from build123d import *

# Parameters (mm, degrees)
SKETCH1_W                = 33
SKETCH1_H                = 33
BOSS_EXTRUDE1_DEPTH      = 33
SKETCH2_W                = 21
SKETCH2_H                = 21
CUT_EXTRUDE1_DEPTH       = 58.15767665
SKETCH3_W                = 21
SKETCH3_H                = 21
CUT_EXTRUDE2_DEPTH       = 58.15767665
SKETCH4_W                = 21
SKETCH4_H                = 21
CUT_EXTRUDE3_DEPTH       = 58.15767665
SKETCH5_R                = 3.05
CUT_EXTRUDE4_DEPTH       = 58.15767665
SKETCH6_R                = 3.05
CUT_EXTRUDE5_DEPTH       = 58.15767665
SKETCH7_R                = 3.05
CUT_EXTRUDE6_DEPTH       = 58.15767665
FILLET1_R                = 6
CHAMFER1_START           = -1
CHAMFER1_OUTLINE_W       = 16
CHAMFER1_OUTLINE_H       = 18
CHAMFER1_DEPTH           = 6.773502692
BOSS_EXTRUDE3_DEPTH      = 8
BOSS_EXTRUDE3_DEPTH_BACK = 10
SKETCH9_W                = 18
SKETCH9_H                = 18
CHAMFER2_SIZE            = 6
FILLET2_R                = 1.25
SKETCH10_R               = 6
BOSS_EXTRUDE4_DEPTH      = 10
SKETCH11_R               = 6
BOSS_EXTRUDE5_DEPTH      = 10
SKETCH12_R               = 6
BOSS_EXTRUDE6_DEPTH      = 10
FILLET3_R                = 2
FILLET4_R                = 2.5


with BuildPart() as part:
    # Sketch1 → Boss-Extrude1 (new body)
    with BuildSketch(Plane(origin=(0, 0, 0), x_dir=(1, 0, 0), z_dir=(0, 1, 0))):
        with Locations((16.5, -16.5)):
            Rectangle(SKETCH1_W, SKETCH1_H)
    extrude(amount=BOSS_EXTRUDE1_DEPTH)

    # Sketch2 → Cut-Extrude1 (cut, through all)
    with BuildSketch(Plane.XY.offset(33)):
        with Locations((22.5, 22.5)):
            Rectangle(SKETCH2_W, SKETCH2_H)
    extrude(amount=-CUT_EXTRUDE1_DEPTH, mode=Mode.SUBTRACT)

    # Sketch3 → Cut-Extrude2 (cut, through all)
    with BuildSketch(Plane.XZ):
        with Locations((22.5, 22.5)):
            Rectangle(SKETCH3_W, SKETCH3_H)
    extrude(amount=-CUT_EXTRUDE2_DEPTH, mode=Mode.SUBTRACT)

    # Sketch4 → Cut-Extrude3 (cut, through all)
    with BuildSketch(Plane.ZY):
        with Locations((22.5, 22.5)):
            Rectangle(SKETCH4_W, SKETCH4_H)
    extrude(amount=-CUT_EXTRUDE3_DEPTH, mode=Mode.SUBTRACT)

    # Sketch5 → Cut-Extrude4 (cut, through all)
    with BuildSketch(Plane.ZY):
        with Locations((27, 6)):
            Circle(SKETCH5_R)
        with Locations((6, 18)):
            Circle(SKETCH5_R)
    extrude(amount=-CUT_EXTRUDE4_DEPTH, mode=Mode.SUBTRACT)

    # Sketch6 → Cut-Extrude5 (cut, through all)
    with BuildSketch(Plane.XZ):
        with Locations(Location((6, 18, 0), (0, 0, 270))):
            Circle(SKETCH6_R)
        with Locations(Location((27, 6, 0), (0, 0, 270))):
            Circle(SKETCH6_R)
    extrude(amount=-CUT_EXTRUDE5_DEPTH, mode=Mode.SUBTRACT)

    # Sketch7 → Cut-Extrude6 (cut, through all)
    with BuildSketch(Plane(origin=(0, 0, 0), x_dir=(-1, 0, 0), z_dir=(0, 0, -1))):
        with Locations((-18, 6)):
            Circle(SKETCH7_R)
        with Locations((-6, 27)):
            Circle(SKETCH7_R)
    extrude(amount=-CUT_EXTRUDE6_DEPTH, mode=Mode.SUBTRACT)

    # Fillet1
    fillet1_edges = [part.edges().sort_by_distance(p)[0] for p in [
        (12, 33, 6),
        (0, 33, 6),
        (6, 12, 33),
        (6, 0, 33),
        (33, 6, 0),
        (33, 6, 12),
    ]]
    fillet(fillet1_edges, radius=FILLET1_R - 0.0001)  # a hair under: the kernel refuses the full size

    # Chamfer1: read off the stored shape, not the designer's step
    # Chamfer1 outline → Chamfer1 (cut)
    with BuildSketch(Plane(origin=(0, 0, 0), x_dir=(0.8164965809277258, -0.40824829046386313, -0.40824829046386313), z_dir=(0.5773502691896258, 0.5773502691896258, 0.5773502691896258)).offset(CHAMFER1_START)):
        with Locations((2, 0)):
            Rectangle(CHAMFER1_OUTLINE_W, CHAMFER1_OUTLINE_H)
    extrude(amount=CHAMFER1_DEPTH, mode=Mode.SUBTRACT)

    # Sketch9 → Boss-Extrude3 (add, two sides: drawn at the far end of the back side and taken through both)
    with BuildSketch(Plane(origin=(0, 0, 0), x_dir=(1, 0, 0), z_dir=(0, 1, 0)).offset(-BOSS_EXTRUDE3_DEPTH_BACK)):
        with Locations((-1, 1)):
            Rectangle(SKETCH9_W, SKETCH9_H)
    extrude(amount=BOSS_EXTRUDE3_DEPTH + BOSS_EXTRUDE3_DEPTH_BACK)

    # Chamfer2
    chamfer2_edges = [part.edges().sort_by_distance(p)[0] for p in [
        (8, -5, 8),
        (8, 8, -5),
        (-5, 8, 8),
    ]]
    chamfer(chamfer2_edges, length=CHAMFER2_SIZE)

    # Fillet2
    # the kernel refuses this fillet: 1.25 mm, written as the material it adds along each edge
    with BuildSketch(Plane(origin=(-4.268829387, 8, 6.268829387), x_dir=(-0.408248290463863, 0.816496580927726, -0.408248290463863), z_dir=(0.7071067811865476, 0, -0.7071067811865476))) as fillet2_piece_1_section:
        with BuildLine():
            CenterArc((FILLET2_R * 1.93185165258, -FILLET2_R), FILLET2_R, 90, 125.264389683)
            Line((FILLET2_R * 1.11535507165, -FILLET2_R * 1.57735026919), (0, 0))
            Line((0, 0), (FILLET2_R * 1.93185165258, 0))
        make_face()
    fillet2_piece_1 = extrude(amount=14.902499954, mode=Mode.PRIVATE)
    fillet2_piece_1 = split(fillet2_piece_1, bisect_by=Plane(origin=(-1.134414693, 11.134414693, 6.268829387), z_dir=(-0.7071067811865476, -0.7071067811865476, 0)), keep=Keep.TOP, mode=Mode.PRIVATE)
    fillet2_piece_1 = split(fillet2_piece_1, bisect_by=Plane(origin=(-4.268829387, 5.865585306, 4.134414694), z_dir=(0, -0.7071067811865476, -0.7071067811865476)), keep=Keep.TOP, mode=Mode.PRIVATE)
    add(fillet2_piece_1)
    with BuildSketch(Plane(origin=(-4.268829387, 6.268829387, 8), x_dir=(-0.4082482904638628, -0.4082482904638628, 0.8164965809277263), z_dir=(0.7071067811865476, -0.7071067811865476, 0))) as fillet2_piece_2_section:
        with BuildLine():
            CenterArc((FILLET2_R * 1.93185165258, FILLET2_R), FILLET2_R, 144.735610317, 125.264389683)
            Line((FILLET2_R * 1.11535507165, FILLET2_R * 1.57735026919), (0, 0))
            Line((0, 0), (FILLET2_R * 1.93185165258, 0))
        make_face()
    fillet2_piece_2 = extrude(amount=14.902499954, mode=Mode.PRIVATE)
    fillet2_piece_2 = split(fillet2_piece_2, bisect_by=Plane(origin=(-4.268829387, 4.134414694, 5.865585306), z_dir=(0, -0.7071067811865476, -0.7071067811865476)), keep=Keep.TOP, mode=Mode.PRIVATE)
    fillet2_piece_2 = split(fillet2_piece_2, bisect_by=Plane(origin=(-1.134414693, 6.268829387, 11.134414693), z_dir=(-0.7071067811865476, 0, -0.7071067811865475)), keep=Keep.TOP, mode=Mode.PRIVATE)
    add(fillet2_piece_2)
    with BuildSketch(Plane(origin=(8, -4.268829387, 6.268829387), x_dir=(0.8164965809277257, -0.40824829046386313, -0.4082482904638633), z_dir=(0, 0.7071067811865476, -0.7071067811865475))) as fillet2_piece_3_section:
        with BuildLine():
            CenterArc((FILLET2_R * 1.93185165258, FILLET2_R), FILLET2_R, 144.735610317, 125.264389683)
            Line((FILLET2_R * 1.11535507165, FILLET2_R * 1.57735026919), (0, 0))
            Line((0, 0), (FILLET2_R * 1.93185165258, 0))
        make_face()
    fillet2_piece_3 = extrude(amount=14.902499954, mode=Mode.PRIVATE)
    fillet2_piece_3 = split(fillet2_piece_3, bisect_by=Plane(origin=(11.134414693, -1.134414693, 6.268829387), z_dir=(-0.7071067811865476, -0.7071067811865476, 0)), keep=Keep.TOP, mode=Mode.PRIVATE)
    fillet2_piece_3 = split(fillet2_piece_3, bisect_by=Plane(origin=(5.865585306, -4.268829387, 4.134414694), z_dir=(-0.7071067811865476, 0, -0.7071067811865475)), keep=Keep.TOP, mode=Mode.PRIVATE)
    add(fillet2_piece_3)

    # Sketch10 → Boss-Extrude4 (add)
    with BuildSketch(Plane.XZ.offset(10)):
        with Locations(Location((-1, -1, 0), (0, 0, 270))):
            Circle(SKETCH10_R)
    extrude(amount=BOSS_EXTRUDE4_DEPTH)

    # Sketch11 → Boss-Extrude5 (add)
    with BuildSketch(Plane.ZY.offset(10)):
        with Locations((-1, -1)):
            Circle(SKETCH11_R)
    extrude(amount=BOSS_EXTRUDE5_DEPTH)

    # Sketch12 → Boss-Extrude6 (add)
    with BuildSketch(Plane(origin=(0, 0, -10), x_dir=(-1, 0, 0), z_dir=(0, 0, -1))):
        with Locations((1, -1)):
            Circle(SKETCH12_R)
    extrude(amount=BOSS_EXTRUDE6_DEPTH)

    # Fillet3
    fillet3_edges = [part.edges().sort_by_distance(p)[0] for p in [
        (8, -4, -10),
        (-4, -10, 8),
        (-10, 8, -4),
        (-10, -1, -10),
        (-4, 8, -10),
        (-10, -4, 8),
        (-10, -10, -1),
        (-1, -10, -10),
        (8, -10, -4),
        (5, -10, 5),
        (5, 5, -10),
        (-10, 5, 5),
    ]]
    fillet(fillet3_edges, radius=FILLET3_R)

    # Fillet4
    fillet4_edges = [part.edges().sort_by_distance(p)[0] for p in [
        (-1, -20, 5),
        (-20, -1, -7),
        (5, -1, -20),
    ]]
    fillet(fillet4_edges, radius=FILLET4_R)


solid = part.part
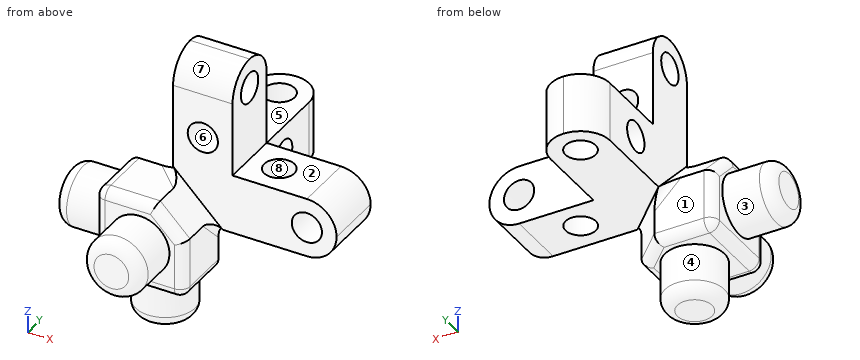
Here's how the part is built. I have some questions about the finished solid (model axes, mm). Face numbers are marked on the shaded views. A direction names the side the tool comes from. Round coordinates to 2 decimals unless told otherwise and drop trailing zeros. Loops run counter-clockwise (first coordinate to the right, second up) from the corner with the lowest first, then second, coordinate; pieces in that order, holes last.
1. If we section it at A-A on y = 18: Write out the boundary of the cut face in (x, z), plus the area to 3 significant figures.
Answer list:
outline: (0, 0) - (12, 0) - (12, 2.95) - (0, 2.95) - close; (0, 9.05) - (12, 9.05) - (12, 12) - (0, 12) - close
area: 70.8 mm2
2. If we section it at B-B on z = 20: Write out the boundary of the cut face in (x, y), plus the area to 3 significant figures.
Answer list:
outline: (0, 0) - (3.7, 0) - (3.7, 12) - (0, 12) - close; (8.3, 0) - (12, 0) - (12, 12) - (8.3, 12) - close
area: 88.7 mm2
3. If we section it at C-C on z = -13: Write out the boundary of the cut face in (x, y).
Answer list:
outline: circle Ø12 at (-1, -1)
4. We'd pull the mould along Z, two halves only. Please class the marked faces 6, 7 and 8: +Z half, -Z half, draft (parallel to the pull), parting line (faces both ways), or undercut.
Answer list:
face 6: undercut
face 7: +Z half
face 8: draft
5. If I drill on line 1 along Y through (x, z) = (6, 3.5); line 2 along Y through (x, z) = (18, 7); line 3 along Y through (x, z) = (8.5, 6), over which ranges is the centre line in solid material (lowest first)?
Answer list:
line 1: y = -9.14 to 16.25, 19.75 to 23.95, 30.05 to 33
line 2: y = 0 to 2.95, 9.05 to 12
line 3: y = 0 to 14.95, 21.05 to 25.25, 28.75 to 32.45
6. Which directions (+Z, -Z, +X, -X, +Y, -Y) give clear straight access to the entire face, cutting with the end or side of a thin tool? Please do the marked faces 1, 2, 3, 4 and 5.
Answer list:
face 1: -Z, -X, +Y
face 2: +Z, +X, +Y, -Y
face 3: -X
face 4: -Z
face 5: +Z, +X, -X, +Y
7. For P1, Ø13, axis at x = 25, z = 7.5, coming from the +Y side; P2, Ø8, axis at x = 1, y = -10, coming from the -Z side; P3, Ø8, axis at x = 6, z = 18, coming from the -Y side, each with a flat end and sliding along its axis, tell me the tip position at first contact or that it passes through.
Answer list:
P1: stops at y = 12
P2: stops at z = -19.31
P3: stops at y = 0
